Can you work these out from the model? Positions are in its coordinate system, mm. Face numbers are marked on the shaded views. A direction names the side the tool comes from. Coordinates: 2 decimals unless noted, no trailing zeros. Loops run counter-clockwise (first coordinate to the right, second up) from the corner with the lowest first, then second, coordinate; pieces in that order, holes last. Notation, with made-up numbers: (-37.75, -39.75) - (9.25, -39.75) arc R8 ccw to (9.25, -25.75) - close; hole circle Ø3 at (73.25, 59). An arc over 180 degrees is marked (long way). Put each result on its own line as item: value. Start each with the question number.
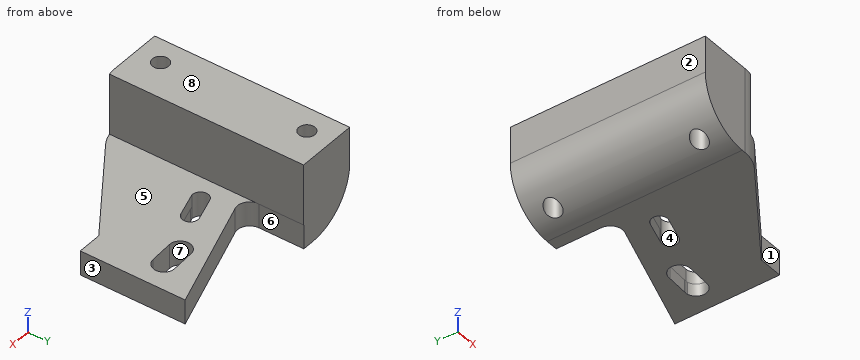
from build123d import *

# Parameters (mm, degrees)
F1_DEPTH     = 80
F2_R         = 3.3
F3_DEPTH     = 25
F5_DEPTH     = 25
F7_W         = 50
F7_H         = 5
F8_DEPTH     = 10
F9_DEPTH     = 25
F11_W        = 20
F11_H        = 80
F11_R        = 3.3
F12_DEPTH    = 30
F13_T1_DEPTH = 180
F15_DEPTH    = 5
F16_DEPTH    = 10
F17_R        = 15


# Not quite as in the source:
# - a fillet or chamfer that OpenCascade refuses, or shapes differently, is made with other operations: its cross-section is extruded or revolved along the edge and cut away or added


with BuildPart() as f1:
    # F0 (on Front) → F1 (new body)
    with BuildSketch(Plane.XZ):
        Polygon((25, 0), (0, 0), (0, -5), (20, -5), (20, -35), (70, -35), (70, -30), (25, -30), align=None)
    extrude(amount=F1_DEPTH)

    # F2 (on face) → F3 (cut)
    with BuildSketch(Plane(origin=(0, 0, -5), x_dir=(1, 0, 0), z_dir=(0, 0, -1))):
        with Locations((10, 70)):
            Circle(F2_R)
        with Locations((10, 10)):
            Circle(F2_R)
    extrude(amount=-F3_DEPTH, mode=Mode.SUBTRACT)

    # F4 (on face) → F5 (cut)
    with BuildSketch(Plane(origin=(0, 0, -35), x_dir=(1, 0, 0), z_dir=(0, 0, -1))):
        Polygon((26.251764968, 80), (70, 50), (70, 80), align=None)
    extrude(amount=-F5_DEPTH, mode=Mode.SUBTRACT)

    # F7 (on face) → F8 (join)
    with BuildSketch(Plane.YZ.offset(70)):
        with Locations((-25, -32.5)):
            Rectangle(F7_W, F7_H)
    extrude(amount=F8_DEPTH)

    # F6 (on face) → F9 (cut)
    with BuildSketch(Plane(origin=(0, 0, -35), x_dir=(1, 0, 0), z_dir=(0, 0, -1))):
        with BuildLine():
            Line((33.2249982655, 32.343756614), (42.1594857766, 29.5393376388))
            Line((42.1594857766, 29.5393376388), (42.9081277459, 29.3043486994))
            ThreePointArc((42.9081277459, 29.3043486994), (46.655005577, 31.7199744818), (44.4654424177, 35.6032919518))
            Line((44.4654424177, 35.6032919518), (35.4531247971, 38.407048043))
            Line((35.4531247971, 38.407048043), (34.4525012517, 38.7183447014))
            ThreePointArc((34.4525012517, 38.7183447014), (30.8539491948, 36.3153921333), (32.8322864897, 32.4670237129))
            Line((32.8322864897, 32.4670237129), (33.2249982655, 32.343756614))
        make_face()
        with BuildLine():
            Line((59.8621358425, 20.2152762479), (68.4127130059, 19.7402941432))
            Line((68.4127130059, 19.7402941432), (69.1118786564, 19.7014556922))
            ThreePointArc((69.1118786564, 19.7014556922), (69.558979499, 19.7364871386), (70, 19.8178952667))
            Line((70, 19.8178952667), (70, 28.1821047333))
            ThreePointArc((70, 28.1821047333), (69.6155307917, 28.2557163727), (69.2259603929, 28.2940589075))
            Line((69.2259603929, 28.2940589075), (59.7544017562, 28.7924677921))
            ThreePointArc((59.7544017562, 28.7924677921), (55.2347672319, 25.0457008651), (58.6655262733, 20.2817475657))
            Line((58.6655262733, 20.2817475657), (59.8621358425, 20.2152762479))
        make_face()
        with BuildLine():
            Line((70, 28.1821047333), (70, 19.8178952667))
            ThreePointArc((70, 19.8178952667), (73.3, 24), (70, 28.1821047333))
        make_face()
    extrude(amount=-F9_DEPTH, mode=Mode.SUBTRACT)

    # F11 (on face) → F12 (join)
    with BuildSketch(Plane(origin=(0, 0, -5), x_dir=(1, 0, 0), z_dir=(0, 0, -1))):
        with Locations((10, 40)):
            Rectangle(F11_W, F11_H)
        with Locations((10, 10)):
            Circle(F11_R, mode=Mode.SUBTRACT)
        with Locations((10, 70)):
            Circle(F11_R, mode=Mode.SUBTRACT)
    extrude(amount=F12_DEPTH)

    # F13: fillet of radius 20 on 1 edges, made by hand

    # F13_s2 → F13_t1 (cut)
    with BuildSketch(Plane.XZ.offset(-50)):
        with BuildLine():
            ThreePointArc((20, -35), (5.8578643763, -29.1421356237), (0, -15))
            Line((0, -15), (0, -35))
            Line((0, -35), (20, -35))
        make_face()
    extrude(amount=F13_T1_DEPTH, mode=Mode.SUBTRACT)

    # F14 (on face) → F15 (join)
    with BuildSketch(Plane.XY.offset(-30)):
        Polygon((80, 0), (25, 0), (25, -80), (26.251764968, -80), (70, -50), (80, -50), (80, -47.8473119438), align=None)
        with BuildLine():
            ThreePointArc((42.9081277459, -29.3043486994), (46.655005577, -31.7199744818), (44.4654424177, -35.6032919518))
            Line((44.4654424177, -35.6032919518), (34.4525012517, -38.7183447014))
            ThreePointArc((34.4525012517, -38.7183447014), (30.8539491948, -36.3153921333), (32.8322864897, -32.4670237129))
            Line((32.8322864897, -32.4670237129), (42.9081277459, -29.3043486994))
        make_face(mode=Mode.SUBTRACT)
        with BuildLine():
            ThreePointArc((69.1118786564, -19.7014556922), (73.2996210658, -23.9429150602), (69.2259603929, -28.2940589075))
            Line((69.2259603929, -28.2940589075), (59.7544017562, -28.7924677921))
            ThreePointArc((59.7544017562, -28.7924677921), (55.2347672319, -25.0457008651), (58.6655262733, -20.2817475657))
            Line((58.6655262733, -20.2817475657), (69.1118786564, -19.7014556922))
        make_face(mode=Mode.SUBTRACT)
    extrude(amount=F15_DEPTH)

    # F10 (on face) → F16 (cut)
    with BuildSketch(Plane(origin=(0, 0, -35), x_dir=(1, 0, 0), z_dir=(0, 0, -1))):
        with BuildLine():
            Line((80, 7), (31.4644035058, 23.1785321647))
            ThreePointArc((31.4644035058, 23.1785321647), (26.9597132524, 22.4913266004), (24.8832646757, 18.4351156745))
            Line((24.8832646757, 18.4351156745), (24.8832646757, 0))
            Line((24.8832646757, 0), (80, 0))
            Line((80, 0), (80, 7))
        make_face()
    extrude(amount=-F16_DEPTH, mode=Mode.SUBTRACT)

    # F17
    f17_edges = [f1.edges().sort_by_distance(p)[0] for p in [
        (26.251765, -80, -30),
    ]]
    fillet(f17_edges, radius=F17_R)


solid = f1.part
Q1. Please list where these lines run through material, in increasing order: line 1 along Y through (x, z) = (10, -13); line 2 along X through (y, z) = (-10, -15); line 3 along Z through (x, y) = (43, -40.5). Write a range as [from, to].
Q2. On a 3-axis mill with a long thin cutter (end or side, diameter ignored), from which of +Z, -Z, +X, -X, +Y, -Y can I reach the whole of each face in a straight line? I mean the marked faces 5, 6, 7 and 8. Say none if no direction works.
Q3. Will these pins go through, and if not, where does the flat tip stop? pin 1 (10 mm diameter, centred on x = 42.5, z = -24.5, fed in from +Y); pin 2 (4 mm diameter, centred on y = -39, z = -8.5, fed in from -X); pin 3 (2 mm diameter, centred on y = -17.5, z = -17.5, fed in from +X); pin 4 (5 mm diameter, centred on x = 73.5, z = -28, fed in from -Y).
Q4. I want a section at A-A on y = -34.5. List the corners of the cut face in (x, z) for me.
Q5. I want a section at D-D on y = -10. List the corners of the cut face in (x, z) for me.
Q6. I want a section at C-C on x = 10. List the corners of the cut face in (y, z) for me, and give its area (3 significant figures).
Q7. I want a section at B-B on z = -11. List the corners of the cut face in (x, y) for me.
Q8. We'd pull the mould along X, two halves only. Please class the marked faces 1, 2, 3 and 4: released by +X, released by -X, zero draft, split by the parting line, or undercut.
Calculated:
1. line 1: [-80, -73.3], [-66.7, -13.3], [-6.7, 0]
1. line 2: [0, 6.7], [13.3, 25]
1. line 3: [-35, -25]
2. face 5: +Z, +X, +Y, -Y
2. face 6: -Z, +Y
2. face 7: +Z, -Z
2. face 8: +Z, +X, -X, +Y, -Y
3. pin 1: y = -17.84
3. pin 2: x = 0
3. pin 3: x = 25
3. pin 4: y = -50
4. outline: (0, -15) arc R20 ccw to (20, -35) - (30.91, -35) - (30.91, -25) - (25, -25) - (25, 0) - (0, 0) - close; (46.06, -35) - (80, -35) - (80, -25) - (46.06, -25) - close
5. outline: (0, -15) arc R20 ccw to (6.7, -29.94) - (6.7, 0) - (0, 0) - close; (13.3, -33.84) arc R20 ccw to (20, -35) - (24.88, -35) - (24.88, -25) - (25, -25) - (25, 0) - (13.3, 0) - close; (71, -35) - (80, -35) - (80, -25) - (71, -25) - close
6. outline: (-80, -32.32) - (-73.3, -32.32) - (-73.3, 0) - (-80, 0) - close; (-66.7, -32.32) - (-13.3, -32.32) - (-13.3, 0) - (-66.7, 0) - close; (-6.7, -32.32) - (0, -32.32) - (0, 0) - (-6.7, 0) - close
6. area: 2,160 mm2
7. outline: (0, -80) - (21.6, -80) arc R15 ccw to (25, -79.61) - (25, 0) - (0, 0) - close; hole circle Ø6.6 at (10, -70); hole circle Ø6.6 at (10, -10)
8. face 1: zero draft
8. face 2: released by -X
8. face 3: released by +X
8. face 4: undercut
